Read the model definition and answer for the solid it produces. Units are mm, in the model's axes. Coordinates: 2 decimals unless noted, no trailing zeros. Return JSON: item names as keys, results as strings. Group by question number.
```python
from build123d import *

# Parameters (mm, degrees)
F1_DEPTH = 1894
F2_R     = 2
F3_R     = 1.99999
F4_W     = 30
F4_H     = 30
F5_DEPTH = 3
F6_W     = 30
F6_H     = 30
F7_DEPTH = 3


# Not quite as in the source:
# - a fillet or chamfer is up to 0.001 mm smaller than in the source, because OpenCascade refuses the exact size


with BuildPart() as f1:
    # F0 (on Top) → F1 (new body)
    with BuildSketch(Plane.XY):
        Polygon((0, 15), (0, 0), (15, 0), (15, 2), (2, 2), (2, 15), align=None)
    extrude(amount=F1_DEPTH)

    # F2
    f2_edges = [f1.edges().sort_by_distance(p)[0] for p in [
        (2, 2, 947),
    ]]
    fillet(f2_edges, radius=F2_R)

    # F3 (radius 2 in the source; OpenCascade refuses exactly that, so slightly less here)
    f3_edges = [f1.edges().sort_by_distance(p)[0] for p in [
        (2, 15, 947),
        (15, 2, 947),
    ]]
    fillet(f3_edges, radius=F3_R)

    # F4 (on face) → F5 (join)
    with BuildSketch(Plane.XY.offset(1894)):
        with Locations((7.5, 7.5)):
            Rectangle(F4_W, F4_H)
    extrude(amount=F5_DEPTH)

    # F6 (on face) → F7 (join)
    with BuildSketch(Plane(origin=(0, 0, 0), x_dir=(1, 0, 0), z_dir=(0, 0, -1))):
        with Locations((7.5, -7.5)):
            Rectangle(F6_W, F6_H)
    extrude(amount=F7_DEPTH)


solid = f1.part
```
1. Given pin 1 (3 mm diameter, centred on y = 8.5, z = 1627.5, fed in from -X); pin 2 (10 mm diameter, centred on x = 10, z = 1017, fed in from +Y); pin 3 (10 mm diameter, centred on y = 9.5, z = 1218, fed in from +X), each flat-ended and moving along its own axis, determine where each tip first touches the part or whether it passes through.
2. For a pull along Z with two mould halves and no side action, classify faces 1 (the face through (7, 8, 1894)), 2 (the face through (7, 7, -3)), 3 (the face through (7, 8, 1897)), 4 (the face through (7, 7, 0)) as released by +Z, released by -Z, zero draft, split by the parting line, or undercut.
3. Straight lines are drawn through the part: L1, parallel to Z at x = 19.75, y = 13.25; L2, parallel to Y at x = 6.25, z = 1129.5. For each, find the intervals that lie inside material, in ascending order.
Result:
{
 "1": {"pin 1": "x = 0", "pin 2": "y = 2", "pin 3": "x = 2"},
 "2": {"face 1": "undercut", "face 2": "released by -Z", "face 3": "released by +Z", "face 4": "undercut"},
 "3": {"L1": "-3 to 0, 1894 to 1897", "L2": "0 to 2"}
}
